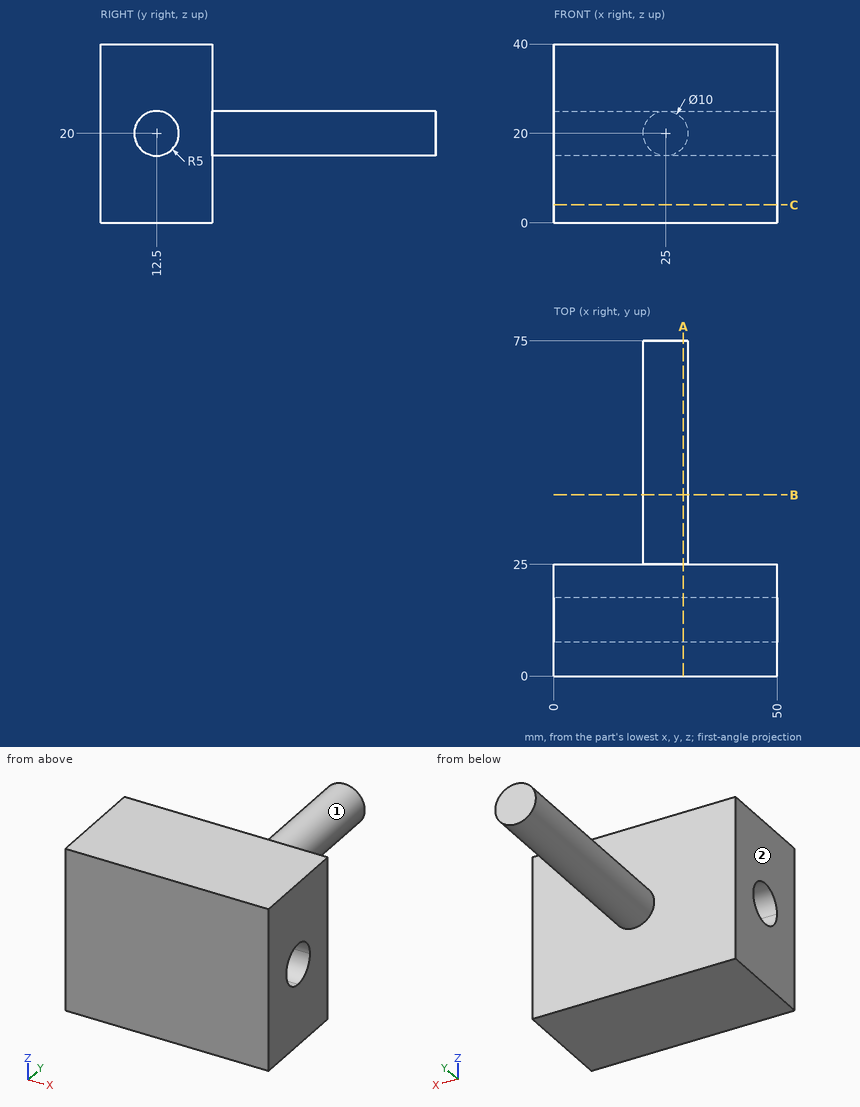
The drawing under review shows one solid part. Ordinate dimensions are in mm from its lowest x, y, z. A direction names the side the tool comes from. Give positions to 0.01 mm unless a question says otherwise; leave off trailing zeros. Loops run counter-clockwise (first coordinate to the right, second up) from the corner with the lowest first, then second, coordinate; pieces in that order, holes last. Notation, with made-up numbers: M 37.25,37 L 58.25,37 A31 ccw 58.25,71 Z; hole C -18.75,57 d11. An arc over 180 degrees is marked long. One line per item, written item: value. Start each with the question number.
Q1. Add section C-C (z = 4). Give the boundary of the cut face in (x, y).
Q2. Clearance check with flat-ended pins moving along their axes: pin 1 Ø6 at (y, z) = (55.5, 23) entering from -X; pin 2 Ø8 at (x, z) = (21.5, 35.5) entering from +Y; pin 3 Ø2 at (y, z) = (50, 22) entering from -X; pin 4 Ø12 at (x, y) = (38.5, 46) entering from -Z. State where each tip first meets the part, or that it passes through.
Q3. Add section B-B (y = 40.5). Give the boundary of the cut face in (x, z).
Q4. Machinability: for the marked faces 1 and 2, which of the approach directions +Z, -Z, +X, -X, +Y, -Y give a long, thin tool a straight path to every point of the face, cutting with its end or side? Answer none if there is none.
Q5. For L1, parallel to Y at x = 14, z = 7.5; L2, parallel to Y at x = 40, z = 16.5; L3, parallel to Z at x = 14, y = 8.5, list the stretches that pass through material, from the lowest coordinate up.
Q6. Add section A-A (x = 29). Give the boundary of the cut face in (y, z).
Reply:
1. outline: M 0,0 L 50,0 L 50,25 L 0,25 Z
2. pin 1: x = 20
2. pin 2: y = 25
2. pin 3: x = 20.1
2. pin 4: through
3. outline: C 25,20 d10
4. face 1: +Y
4. face 2: +Z, -Z, -X, +Y, -Y
5. L1: 0 to 25
5. L2: 0 to 8.93, 16.07 to 25
5. L3: 0 to 17, 23 to 40
6. outline: M 0,0 L 25,0 L 25,17 L 75,17 L 75,23 L 25,23 L 25,40 L 0,40 Z; hole C 12.5,20 d10
